from build123d import *

# Parameters (mm, degrees)
SKETCH1_W           = 19.812
SKETCH1_H           = 40
BOSS_EXTRUDE1_DEPTH = 3.175
FILLET2_R           = 2.54


with BuildPart() as part:
    # Sketch1 → Boss-Extrude1 (new body)
    with BuildSketch(Plane.XY):
        Polygon((12.7, 0), (50.8, 0), (50.8, 38.1), (50.8, 57.15), (9.525, 57.15), (9.525, 38.1), (9.525, 22.184785263), (6.35, 22.184785263), (6.35, 38.1), (0, 38.1), (0, 9.525), (12.7, 9.525), align=None)
        with Locations((34.925, 32.177185263)):
            Rectangle(SKETCH1_W, SKETCH1_H, mode=Mode.SUBTRACT)
    extrude(amount=BOSS_EXTRUDE1_DEPTH)

    # Fillet2
    fillet2_edges = [part.edges().sort_by_distance(p)[0] for p in [
        (50.8, 0, 1.5875),
        (0, 9.525, 1.5875),
        (0, 38.1, 1.5875),
        (6.35, 38.1, 1.5875),
        (9.525, 57.15, 1.5875),
        (50.8, 57.15, 1.5875),
    ]]
    fillet(fillet2_edges, radius=FILLET2_R)


solid = part.part
Source: CAD feature listing. Evaluate the final solid. Frame: model axes, mm. A direction names the side the tool comes from. Give positions to 0.01 mm unless a question says otherwise; leave off trailing zeros. Write each loop counter-clockwise with the first axis right and the second up, starting at its lowest first coordinate (ties: lowest second). Pieces come first, ordered by that corner, then holes. Notation, with made-up numbers: M 24.5,47 L 71.5,47 A29 cw 71.5,74 Z; hole C 60.25,23 d5. An arc over 180 degrees is marked long. Return JSON: item names as keys, results as strings. Group by question number.
1) Ray query, L1, parallel to X at y = 24, z = 2.7 (3 decimals); L2, parallel to Y at x = 35.5, z = 1.3; L3, parallel to X at y = 48, z = 0.95 (3 decimals). Return the intervals inside material, ascending.
2) Draft query along Y for faces 1 (the face through (9.525, 39, 2)), 2 (the face through (25.019, 32, 2)), 3 (the face through (8, 22.185, 2)). Return one class per face: released by +Y, released by -Y, zero draft, split by the parting line, or undercut.
3) First-contact query: pin 1 Ø1.4 at (x, z) = (3, 2) entering from +Y; pin 2 Ø1.6 at (y, z) = (3, 2) entering from -X; pin 3 Ø4 at (x, y) = (10.5, 38.5) entering from -Z; pin 4 Ø1 at (x, z) = (7.5, 2) entering from -Y (3 decimals). Flat tips, straight axial feed; report the tip coordinate or a pass-through.
4) Cut plane D-D, the plane y = 23. Output: boundary loops of the cut face in (x, z) (3 decimals).
5) Cut plane A-A, the plane x = 27.5. Output: boundary loops of the cut face in (y, z) (3 decimals), then the cut area to 3 significant figures.
6) Set-up query: faces 4 (the face through (3, 38.1, 2)), 5 (the face through (19, 29, 3.175)), 6 (the face through (35, 52.177, 2)), 7 (the face through (12.7, 5, 2)), 8 (the face through (5.586, 37.376, 1.61)). Return all of +Z, -Z, +X, -X, +Y, -Y with unobstructed straight access to the full face (end or side cutting, diameter ignored); none if empty.
7) Cut plane B-B, the plane y = 15. Output: boundary loops of the cut face in (x, z) (3 decimals).
8) Cut plane C-C, the plane z = 2.15. Output: boundary loops of the cut face in (x, y) (3 decimals).
Data:
{
 "1": {"L1": "x = 0 to 6.35, 9.525 to 25.019, 44.831 to 50.8", "L2": "y = 0 to 12.18, 52.18 to 57.15", "L3": "x = 9.525 to 25.019, 44.831 to 50.8"},
 "2": {"face 1": "zero draft", "face 2": "undercut", "face 3": "released by +Y"},
 "3": {"pin 1": "stops at y = 38.1", "pin 2": "stops at x = 12.7", "pin 3": "stops at z = 0", "pin 4": "stops at y = 9.525"},
 "4": {"outline": "M 0,0 L 6.35,0 L 6.35,3.175 L 0,3.175 Z; M 9.525,0 L 25.019,0 L 25.019,3.175 L 9.525,3.175 Z; M 44.831,0 L 50.8,0 L 50.8,3.175 L 44.831,3.175 Z"},
 "5": {"outline": "M 0,0 L 12.177,0 L 12.177,3.175 L 0,3.175 Z; M 52.177,0 L 57.15,0 L 57.15,3.175 L 52.177,3.175 Z", "area": "54.5 mm²"},
 "6": {"face 4": "+Z, -Z, -X, +Y", "face 5": "+Z, +X, -X, +Y, -Y", "face 6": "+Z, -Z", "face 7": "+Z, -Z, -X, -Y", "face 8": "+Z, -Z, +Y"},
 "7": {"outline": "M 0,0 L 25.019,0 L 25.019,3.175 L 0,3.175 Z; M 44.831,0 L 50.8,0 L 50.8,3.175 L 44.831,3.175 Z"},
 "8": {"outline": "M 0,12.065 A2.54 ccw 2.54,9.525 L 12.7,9.525 L 12.7,0 L 48.26,0 A2.54 ccw 50.8,2.54 L 50.8,54.61 A2.54 ccw 48.26,57.15 L 12.065,57.15 A2.54 ccw 9.525,54.61 L 9.525,22.185 L 6.35,22.185 L 6.35,35.56 A2.54 ccw 3.81,38.1 L 2.54,38.1 A2.54 ccw 0,35.56 Z; hole M 25.019,12.177 L 44.831,12.177 L 44.831,52.177 L 25.019,52.177 Z"}
}
